```python
from build123d import *

# Parameters (mm, degrees)
F0_R      = 67
F1_DEPTH  = 2.5
F2_R      = 64.375
F2_R_2    = 62.625
F3_DEPTH  = 5
F4_R      = 62.625
F4_R_2    = 58.875
F5_DEPTH  = 5
F6_R      = 4.75
F6_R_2    = 5.75
F6_R_3    = 2.1
F7_DEPTH  = 5.001
F8_R      = 5.25
F8_R_2    = 4.75
F9_DEPTH  = 0.5
F8_R_3    = 6.25
F8_R_4    = 5.75
F10_DEPTH = 1
F8_R_5    = 2.1
F11_DEPTH = 3
F12_R     = 6.25
F12_R_2   = 5.75
F13_DEPTH = 1
F14_W     = 5
F14_H     = 12
F15_DEPTH = 1.5
F16_COUNT = 6
F16_ANGLE = 150
F17_COUNT = 6
F17_ANGLE = 150


with BuildPart() as f1:
    # F0 (on Top) → F1 (new body, symmetric)
    with BuildSketch(Plane.XY):
        Circle(F0_R)
    extrude(amount=F1_DEPTH, both=True)

    # F2 (on Top) → F3 (join)
    with BuildSketch(Plane.XY):
        Circle(F2_R)
        Circle(F2_R_2, mode=Mode.SUBTRACT)
    extrude(amount=F3_DEPTH)

    # F4 (on Top) → F5 (cut)
    with BuildSketch(Plane.XY):
        Circle(F4_R)
        Circle(F4_R_2, mode=Mode.SUBTRACT)
    extrude(amount=F5_DEPTH, mode=Mode.SUBTRACT)

    # F6 (on face) → F7 (cut, through all)
    with BuildSketch(Plane.XY.offset(2.5)):
        Circle(F6_R)
        with Locations((0, 18.75)):
            Circle(F6_R_2)
        with Locations((0, 46.25)):
            Circle(F6_R_2)
        with Locations((17.5, -8)):
            Circle(F6_R_3)
        with Locations((-17.5, -8)):
            Circle(F6_R_3)
    extrude(amount=-F7_DEPTH, mode=Mode.SUBTRACT)

    # F8 (on face) → F9 (cut)
    with BuildSketch(Plane.XY.offset(2.5)):
        Circle(F8_R)
        Circle(F8_R_2, mode=Mode.SUBTRACT)
    extrude(amount=-F9_DEPTH, mode=Mode.SUBTRACT)

    # F8 (on face) → F10 (cut)
    with BuildSketch(Plane.XY.offset(2.5)):
        with Locations((0, 18.75)):
            Circle(F8_R_3)
        with Locations((0, 18.75)):
            Circle(F8_R_4, mode=Mode.SUBTRACT)
        with Locations((0, 46.25)):
            Circle(F8_R_3)
        with Locations((0, 46.25)):
            Circle(F8_R_4, mode=Mode.SUBTRACT)
    extrude(amount=-F10_DEPTH, mode=Mode.SUBTRACT)

    # F8 (on face) → F11 (cut)
    with BuildSketch(Plane.XY.offset(2.5)):
        Polygon((17.5327657222, -12.3300030494), (21.2662755003, -10.1366255769), (21.2335097781, -5.8066225275), (17.4672342778, -3.6699969506), (13.7337244997, -5.8633744231), (13.7664902219, -10.1933774725), align=None)
        with Locations((17.5, -8)):
            Circle(F8_R_5, mode=Mode.SUBTRACT)
        Polygon((-17.4672342778, -12.3300030494), (-13.7337244997, -10.1366255769), (-13.7664902219, -5.8066225275), (-17.5327657222, -3.6699969506), (-21.2662755003, -5.8633744231), (-21.2335097781, -10.1933774725), align=None)
        with Locations((-17.5, -8)):
            Circle(F8_R_5, mode=Mode.SUBTRACT)
    extrude(amount=-F11_DEPTH, mode=Mode.SUBTRACT)

    # F12 (on face) → F13 (cut)
    with BuildSketch(Plane(origin=(0, 0, -2.5), x_dir=(1, 0, 0), z_dir=(0, 0, -1))):
        with Locations((0, -46.25)):
            Circle(F12_R)
        with Locations((0, -46.25)):
            Circle(F12_R_2, mode=Mode.SUBTRACT)
        with Locations((0, -18.75)):
            Circle(F12_R)
        with Locations((0, -18.75)):
            Circle(F12_R_2, mode=Mode.SUBTRACT)
    extrude(amount=-F13_DEPTH, mode=Mode.SUBTRACT)

    # F14 (on face) → F15 (join)
    with BuildSketch(Plane.XY.offset(2.5)):
        with Locations((0, -50)):
            Rectangle(F14_W, F14_H)
    f15 = extrude(amount=F15_DEPTH)

    # F16: F15 ×6 about axis
    f16_axis = Axis((0, 0, 2.5), (0, 0, -1))
    for i in range(1, F16_COUNT):
        add(f15.rotate(f16_axis, i * F16_ANGLE / (F16_COUNT - 1)))

    # F17: F15 ×6 about axis
    f17_axis = Axis((0, 0, 2.5), (0, 0, 1))
    for i in range(1, F17_COUNT):
        add(f15.rotate(f17_axis, i * F17_ANGLE / (F17_COUNT - 1)))


solid = f1.part
```
Verification items for the finished model (mm, model axes). A direction names the side the tool comes from. Round coordinates to 2 decimals unless told otherwise and drop trailing zeros. Order: outer loops, then holes, each group sorted by start corner. A loop starts at its lowest first (then second) coordinate and runs counter-clockwise, first axis right, second up.
1) Depth check by flat-ended pin: pin 1 (3 mm diameter, centred on x = 7.5, y = 31.5, fed in from +Z); pin 2 (3 mm diameter, centred on y = -15, z = 1.5, fed in from +X); pin 3 (3 mm diameter, centred on x = -41, y = -25, fed in from +Z); pin 4 (10 mm diameter, centred on x = 0, y = 18.75, fed in from -Z). Enter the tip coordinate at first touch or a pass-through.
Geometry says:
pin 1: stops at z = 2.5
pin 2: stops at x = 65.63
pin 3: stops at z = 4
pin 4: passes through
2) Cross-section at C-C, the plane x = 41. Record the cut outline in (y, z).
Geometry says:
outline: (-52.99, -2.5) - (52.99, -2.5) - (52.99, 2.5) - (49.63, 2.5) - (49.63, 5) - (47.34, 5) - (47.34, 0) - (42.25, 0) - (42.25, 2.5) - (26.56, 2.5) - (26.56, 4) - (20.78, 4) - (20.78, 2.5) - (-20.78, 2.5) - (-20.78, 4) - (-26.56, 4) - (-26.56, 2.5) - (-42.25, 2.5) - (-42.25, 0) - (-47.34, 0) - (-47.34, 5) - (-49.63, 5) - (-49.63, 2.5) - (-52.99, 2.5) - close
3) Draft check along X on faces 4 (the cylindrical face through (5, 1.6, 2.3)), 5 (the cylindrical face through (-13.955, -62.844, 3.732)). Enter one of: +X half, -X half, draft (parallel to the pull), parting line (faces both ways), or undercut.
Geometry says:
face 4: undercut
face 5: parting line
4) Tool access check on faces 1 (the flat face through (-27.207, 42.124, 3.24)), 2 (the cylindrical face through (2.192, -4.214, -0.219)), 3 (the flat face through (3, 24, -1.5)). Record the directions out of +Z, -Z, +X, -X, +Y, -Y that give a thin tool (end or side, any length) a straight path to the whole face; none if there is none.
Geometry says:
face 1: +Z
face 2: +Z, -Z
face 3: -Z
5) Cross-section at B-B, the plane x = 0. Give the number of separate pieces and of enclosed holes in the cut face, plus the area to 3 significant figures.
Geometry says:
separate pieces: 4
enclosed holes: 0
area: 511 mm2
6) Material ranges on line 1 (Y direction, x = 0, z = 1) (3 decimals); line 2 (X direction, y = 16, z = 2.25); line 3 (Y direction, x = -30, z = 3), recorded low to high.
Geometry says:
line 1: y = -67 to -62.625, -58.875 to -4.75, 4.75 to 13, 24.5 to 40.5, 52 to 58.875, 62.625 to 67
line 2: x = -65.06 to -60.55, -56.66 to -5.61, 5.61 to 56.66, 60.55 to 65.06
line 3: y = -56.96 to -54.97, -47.34 to -46.96, 46.96 to 47.34, 54.97 to 56.96
